Read the model definition and answer for the solid it produces. Units are mm, in the model's axes. A direction names the side the tool comes from. Coordinates: 2 decimals unless noted, no trailing zeros. Order: outer loops, then holes, each group sorted by start corner. A loop starts at its lowest first (then second) coordinate and runs counter-clockwise, first axis right, second up. Notation, with made-up numbers: (53, -23.5) -> (109, -23.5) arc R3 ccw to (109, -18.5) -> close; hole circle Ø3 at (58, -7). An arc over 180 degrees is marked (long way). Use CSV: the item, a comma, the result in double quotes.
```python
from build123d import *

# Parameters (mm, degrees)
FEMALE_MATING_FOOT_VERIFY_START                = 34.6
SKETCH_1_W                                     = 58.4
SKETCH_1_H                                     = 11.9
FEMALE_MATING_FOOT_VERIFY_DEPTH                = 3.4
RIGHT_ANGLE_SOCKET_INFERRED_NOT_CERTIFIE_START = 38
SKETCH_2_W                                     = 58.4
SKETCH_2_H                                     = 3.4
RIGHT_ANGLE_SOCKET_INFERRED_NOT_CERTIFIE_DEPTH = 12


with BuildPart() as part:
    # 草图1 → Female_mating_foot_VERIFY (new body)
    with BuildSketch(Plane.XY.offset(FEMALE_MATING_FOOT_VERIFY_START)):
        with Locations((0, -135.95)):
            Rectangle(SKETCH_1_W, SKETCH_1_H)
    extrude(amount=FEMALE_MATING_FOOT_VERIFY_DEPTH)

    # 草图2 → Right_angle_socket_INFERRED_NOT_CERTIFIED (add)
    with BuildSketch(Plane.XY.offset(RIGHT_ANGLE_SOCKET_INFERRED_NOT_CERTIFIE_START)):
        with Locations((0, -131.7)):
            Rectangle(SKETCH_2_W, SKETCH_2_H)
    extrude(amount=RIGHT_ANGLE_SOCKET_INFERRED_NOT_CERTIFIE_DEPTH)


solid = part.part
```
Item 1: Straight lines are drawn through the part: line 1 along Y through (x, z) = (-11.5, 38.25); line 2 along Z through (x, y) = (-24.5, -133.75). For each, find the intervals that lie inside material, in ascending order.
Return value:
line 1,"y = -133.4 to -130"
line 2,"z = 34.6 to 38"
Item 2: A tool of negligible diameter and unlimited length cuts with its end or side. For faces 1 (the flat face through (0, -133.4, 44)), 2 (the flat face through (-29.2, -133, 40)), from which of +Z, -Z, +X, -X, +Y, -Y can it reach the whole face along a straight path? Write none if from no direction.
Return value:
face 1,"+Z, +X, -X, -Y"
face 2,"+Z, -Z, -X, +Y, -Y"
Item 3: Find section B-B, the plane z = 44.5. Give the vertices of the cut face in (x, y).
Return value:
outline,"(-29.2, -133.4) -> (29.2, -133.4) -> (29.2, -130) -> (-29.2, -130) -> close"
Item 4: Find section C-C, the plane y = -139. Give the vertices of the cut face in (x, z), then the cut area to 3 significant figures.
Return value:
outline,"(-29.2, 34.6) -> (29.2, 34.6) -> (29.2, 38) -> (-29.2, 38) -> close"
area,"199 mm^2"
Item 5: Find section A-A, the plane x = 20.5. Give the vertices of the cut face in (y, z), then the cut area to 3 significant figures.
Return value:
outline,"(-141.9, 34.6) -> (-130, 34.6) -> (-130, 50) -> (-133.4, 50) -> (-133.4, 38) -> (-141.9, 38) -> close"
area,"81.3 mm^2"
